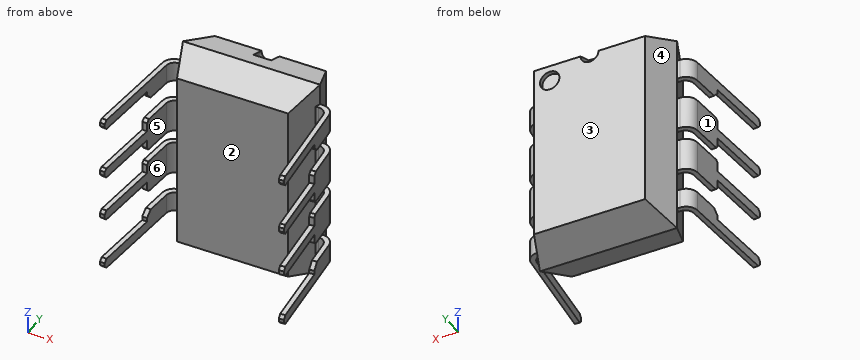
from build123d import *

# Parameters (mm, degrees)
BOSS_EXTRUDE1_DEPTH     = 9.5
CUT_EXTRUDE2_DEPTH      = 9.5
CUT_EXTRUDE2_DEPTH_BACK = 9.5
CUT_EXTRUDE3_DEPTH      = 0.7
SKETCH4_W               = 0.83
SKETCH4_H               = 0.7
CUT_EXTRUDE4_DEPTH      = 0.7
BOSS_EXTRUDE2_START     = -0.762
BOSS_EXTRUDE2_DEPTH     = 0.912
CUT_EXTRUDE5_DEPTH      = 10.15
SKETCH9_R               = 0.45
CUT_EXTRUDE7_DEPTH      = 0.2
BOSS_EXTRUDE3_DEPTH     = 0.762
CUT_EXTRUDE6_DEPTH      = 0.762
MIRROR2_START           = -0.762
MIRROR2_COPY_1_DEPTH    = 0.912
MIRROR2_COPY_2_DEPTH    = 10.15
MIRROR2_COPY_3_DEPTH    = 0.762
MIRROR2_COPY_4_DEPTH    = 0.762


with BuildPart() as part:
    # Sketch1 → Boss-Extrude1 (new body)
    with BuildSketch(Plane.XY):
        Polygon((-24.934327538, -0.557710036), (-25.534514454, 1.091289964), (-30.684140621, 1.091289964), (-31.284327538, -0.557710036), (-30.683412681, -2.208710036), (-25.535242395, -2.208710036), align=None)
    extrude(amount=-BOSS_EXTRUDE1_DEPTH)

    # Sketch2 → Cut-Extrude2 (cut, two sides)
    with BuildSketch(Plane(origin=(-30.683898403, -0.0067685, 0), x_dir=(0, 0, 1), z_dir=(-0.9999999756704636, -0.00022058801540043594, 0))) as cut_extrude2_sk:
        Polygon((-0.616330332, -2.245563479), (0, -0.552209808), (0, -2.212209808), align=None)
        Polygon((-0.60064854, 1.098058491), (0, -0.552209808), (0, 1.098058491), align=None)
        Polygon((-9.5, -2.212209808), (-8.892247033, -2.221997362), (-9.5, -0.552209808), align=None)
        Polygon((-9.5, -0.552209808), (-9.5, 1.098058491), (-8.89935146, 1.098058491), align=None)
    extrude(amount=CUT_EXTRUDE2_DEPTH, mode=Mode.SUBTRACT)
    extrude(cut_extrude2_sk.sketch, amount=-CUT_EXTRUDE2_DEPTH_BACK, mode=Mode.SUBTRACT)

    # Sketch3 → Cut-Extrude3 (cut)
    with BuildSketch(Plane(origin=(0, 1.091289964, 0), x_dir=(1, 0, 0), z_dir=(0, 1, 0))):
        with BuildLine():
            Line((-28.524327536, 0.600475134), (-27.694327539, 0.600408495))
            ThreePointArc((-27.694327539, 0.600408495), (-28.109294218, 1.015441813), (-28.524327536, 0.600475134))
        make_face()
    extrude(amount=-CUT_EXTRUDE3_DEPTH, mode=Mode.SUBTRACT)

    # Sketch4 → Cut-Extrude4 (cut)
    with BuildSketch(Plane(origin=(4.8027e-05, 0, -0.598184984), x_dir=(-0.9999999967769609, 0, -8.028747138262029e-05), z_dir=(8.028747138262029e-05, 0, -0.9999999967769609))):
        with Locations((28.109375655, 0.741289964)):
            Rectangle(SKETCH4_W, SKETCH4_H)
    extrude(amount=-CUT_EXTRUDE4_DEPTH, mode=Mode.SUBTRACT)


with BuildPart() as boss_extrude2_tool:
    # Sketch5 → Boss-Extrude2 (new body)
    with BuildSketch(Plane.XY.offset(-1.143).offset(BOSS_EXTRUDE2_START)):
        with BuildLine():
            Line((-24.934327536, -0.557713614), (-24.80305479, -0.557713614))
            ThreePointArc((-24.80305479, -0.557713614), (-24.431480176, -0.702211079), (-24.255147706, -1.059777956))
            Line((-24.255147706, -1.059777956), (-23.8457982, -5.738664215))
            Line((-23.8457982, -5.738664215), (-24.074922981, -5.758710036))
            Line((-24.074922981, -5.758710036), (-24.477883405, -1.152851317))
            ThreePointArc((-24.477883405, -1.152851317), (-24.606125201, -0.892802679), (-24.876361284, -0.787713614))
            Line((-24.876361284, -0.787713614), (-25.018040872, -0.787713614))
            Line((-25.018040872, -0.787713614), (-24.934327536, -0.557713614))
        make_face()
    boss_extrude2 = extrude(amount=BOSS_EXTRUDE2_DEPTH)


with BuildPart() as part_1:
    add(part.part)


with BuildPart() as part_2:
    # Boss-Extrude2: joined with boss_extrude2_tool
    add(part_1.part.fuse(boss_extrude2_tool.part, tol=0.00001))

    # Sketch6 → Cut-Extrude5 (cut)
    with BuildSketch(Plane(origin=(-24.162916864, -2.113981303, 0), x_dir=(0, 0, -1), z_dir=(0.9961946980917458, 0.08715574274765556, 0))):
        Polygon((0.993, -3.502234692), (0.993, -3.638528611), (1.129293919, -3.638528611), align=None)
        Polygon((1.449, -3.502234692), (1.292810168, -3.638528611), (1.449, -3.638528611), align=None)
        Polygon((1.449, -3.502234692), (1.449, -3.638528611), (1.905, -3.638528611), (1.905, -0.186528611), (1.628, -0.463528611), (1.449, -0.463528611), align=None)
    cut_extrude5 = extrude(amount=-CUT_EXTRUDE5_DEPTH, mode=Mode.SUBTRACT)

    # Sketch9 → Cut-Extrude7 (cut)
    with BuildSketch(Plane(origin=(0, 1.091289964, 0), x_dir=(1, 0, 0), z_dir=(0, 1, 0))):
        with Locations(Location((-26.264514454, 1.330293701, 0), (0, 0, 180))):
            Circle(SKETCH9_R)
    extrude(amount=-CUT_EXTRUDE7_DEPTH, mode=Mode.SUBTRACT)

    # Sketch7 → Boss-Extrude3 (add, symmetric)
    with BuildSketch(Plane.XY.offset(-3.683)):
        with BuildLine():
            Line((-24.934327538, -0.557710036), (-24.803054792, -0.557710036))
            ThreePointArc((-24.803054792, -0.557710036), (-24.431480177, -0.7022075), (-24.255147708, -1.059774377))
            Line((-24.255147708, -1.059774377), (-23.845798202, -5.738660636))
            Line((-23.845798202, -5.738660636), (-24.074922983, -5.758706457))
            Line((-24.074922983, -5.758706457), (-24.477883406, -1.152847739))
            ThreePointArc((-24.477883406, -1.152847739), (-24.606125202, -0.892799101), (-24.876361286, -0.787710036))
            Line((-24.876361286, -0.787710036), (-25.018040873, -0.787710036))
            Line((-25.018040873, -0.787710036), (-24.934327538, -0.557710036))
        make_face()
    boss_extrude3 = extrude(amount=BOSS_EXTRUDE3_DEPTH, both=True)

    # Sketch8 → Cut-Extrude6 (cut)
    with BuildSketch(Plane(origin=(-24.162916555, -2.113981276, 0), x_dir=(0, 0, -1), z_dir=(0.9961946980917459, 0.08715574274765502, 0))):
        Polygon((2.921, -3.638525046), (3.4545, -3.638525046), (3.4545, -3.512139824), (3.4545, -0.463528611), (3.048, -0.463528611), (2.921, -0.309075706), align=None)
        Polygon((3.9115, -0.463528611), (3.9115, -3.512139824), (3.9115, -3.638525046), (4.445, -3.638525046), (4.445, -0.359101958), (4.318, -0.463528611), align=None)
        Polygon((3.4545, -3.512139824), (3.4545, -3.638525046), (3.558421148, -3.638525046), align=None)
        Polygon((3.9115, -3.512139824), (3.757794765, -3.638525046), (3.9115, -3.638525046), align=None)
    cut_extrude6 = extrude(amount=-CUT_EXTRUDE6_DEPTH, mode=Mode.SUBTRACT)

    # Mirror1: Boss-Extrude2, Cut-Extrude5, Boss-Extrude3, Cut-Extrude6 across plane
    add(boss_extrude2.mirror(Plane.XY.offset(-4.75)))
    add(cut_extrude5.mirror(Plane.XY.offset(-4.75)), mode=Mode.SUBTRACT)
    add(boss_extrude3.mirror(Plane.XY.offset(-4.75)))
    add(cut_extrude6.mirror(Plane.XY.offset(-4.75)), mode=Mode.SUBTRACT)

    # Mirror2: Boss-Extrude2, Cut-Extrude5, Boss-Extrude3, Cut-Extrude6 across plane
    add(boss_extrude2.mirror(Plane(origin=(-28.109327538, 0, 0), x_dir=(0, 0, 1), z_dir=(1, 0, 0))))
    add(cut_extrude5.mirror(Plane(origin=(-28.109327538, 0, 0), x_dir=(0, 0, 1), z_dir=(1, 0, 0))), mode=Mode.SUBTRACT)
    add(boss_extrude3.mirror(Plane(origin=(-28.109327538, 0, 0), x_dir=(0, 0, 1), z_dir=(1, 0, 0))))
    add(cut_extrude6.mirror(Plane(origin=(-28.109327538, 0, 0), x_dir=(0, 0, 1), z_dir=(1, 0, 0))), mode=Mode.SUBTRACT)


with BuildPart() as mirror2_copy_1_tool:
    # Mirror2 copy 1 sketch → Mirror2 copy 1 (new body)
    with BuildSketch(Plane(origin=(-56.218655076, 0, -8.357), x_dir=(-1, 0, 0), z_dir=(0, 0, -1)).offset(MIRROR2_START)):
        with BuildLine():
            Line((-24.934327536, -0.557713614), (-24.80305479, -0.557713614))
            ThreePointArc((-24.80305479, -0.557713614), (-24.431480176, -0.702211079), (-24.255147706, -1.059777956))
            Line((-24.255147706, -1.059777956), (-23.8457982, -5.738664215))
            Line((-23.8457982, -5.738664215), (-24.074922981, -5.758710036))
            Line((-24.074922981, -5.758710036), (-24.477883405, -1.152851317))
            ThreePointArc((-24.477883405, -1.152851317), (-24.606125201, -0.892802679), (-24.876361284, -0.787713614))
            Line((-24.876361284, -0.787713614), (-25.018040872, -0.787713614))
            Line((-25.018040872, -0.787713614), (-24.934327536, -0.557713614))
        make_face()
    extrude(amount=MIRROR2_COPY_1_DEPTH)


with BuildPart() as part_3:
    add(part_2.part)


with BuildPart() as part_4:
    # Mirror2 copy 1: joined with mirror2_copy_1_tool
    add(part_3.part.fuse(mirror2_copy_1_tool.part, tol=0.00001))

    # Mirror2 copy 2 sketch → Mirror2 copy 2 (cut)
    with BuildSketch(Plane(origin=(-32.055738211, -2.113981303, -9.5), x_dir=(0, 0, 1), z_dir=(-0.9961946980917458, 0.08715574274765556, 0))):
        Polygon((0.993, -3.502234692), (0.993, -3.638528611), (1.129293919, -3.638528611), align=None)
        Polygon((1.449, -3.502234692), (1.292810168, -3.638528611), (1.449, -3.638528611), align=None)
        Polygon((1.449, -3.502234692), (1.449, -3.638528611), (1.905, -3.638528611), (1.905, -0.186528611), (1.628, -0.463528611), (1.449, -0.463528611), align=None)
    extrude(amount=-MIRROR2_COPY_2_DEPTH, mode=Mode.SUBTRACT)

    # Mirror2 copy 3 sketch → Mirror2 copy 3 (add, symmetric)
    with BuildSketch(Plane(origin=(-56.218655076, 0, -5.817), x_dir=(-1, 0, 0), z_dir=(0, 0, -1))):
        with BuildLine():
            Line((-24.934327538, -0.557710036), (-24.803054792, -0.557710036))
            ThreePointArc((-24.803054792, -0.557710036), (-24.431480177, -0.7022075), (-24.255147708, -1.059774377))
            Line((-24.255147708, -1.059774377), (-23.845798202, -5.738660636))
            Line((-23.845798202, -5.738660636), (-24.074922983, -5.758706457))
            Line((-24.074922983, -5.758706457), (-24.477883406, -1.152847739))
            ThreePointArc((-24.477883406, -1.152847739), (-24.606125202, -0.892799101), (-24.876361286, -0.787710036))
            Line((-24.876361286, -0.787710036), (-25.018040873, -0.787710036))
            Line((-25.018040873, -0.787710036), (-24.934327538, -0.557710036))
        make_face()
    extrude(amount=MIRROR2_COPY_3_DEPTH, both=True)

    # Mirror2 copy 4 sketch → Mirror2 copy 4 (cut)
    with BuildSketch(Plane(origin=(-32.055738521, -2.113981276, -9.5), x_dir=(0, 0, 1), z_dir=(-0.9961946980917459, 0.08715574274765502, 0))):
        Polygon((2.921, -3.638525046), (3.4545, -3.638525046), (3.4545, -3.512139824), (3.4545, -0.463528611), (3.048, -0.463528611), (2.921, -0.309075706), align=None)
        Polygon((3.9115, -0.463528611), (3.9115, -3.512139824), (3.9115, -3.638525046), (4.445, -3.638525046), (4.445, -0.359101958), (4.318, -0.463528611), align=None)
        Polygon((3.4545, -3.512139824), (3.4545, -3.638525046), (3.558421148, -3.638525046), align=None)
        Polygon((3.9115, -3.512139824), (3.757794765, -3.638525046), (3.9115, -3.638525046), align=None)
    extrude(amount=-MIRROR2_COPY_4_DEPTH, mode=Mode.SUBTRACT)


solid = part_4.part
Source: CAD feature listing. Evaluate the final solid. Frame: model axes, mm. Face numbers are marked on the shaded views. A direction names the side the tool comes from. Round coordinates to 2 decimals unless told otherwise and drop trailing zeros. Loops run counter-clockwise (first coordinate to the right, second up) from the corner with the lowest first, then second, coordinate; pieces in that order, holes last. Notation, with made-up numbers: (88, 14.5) - (145, 14.5) arc R28 cw to (145, 42.5) - close; hole circle Ø8 at (89, 55). An arc over 180 degrees is marked (long way). Write item = value, one per line. Start each with the question number.
Item 1: Mould query, pull axis X, two halves, no side actions, for the marked faces 3, 4, 5 and 6. Classes: released by +X, released by -X, zero draft, split by the parting line, or undercut.
Item 2: Section query A-A on y = -4.25. Count the separate pieces of the cut face and the enclosed holes in it, plus the area to 3 significant figures.
Item 3: First-contact query: pin 1 Ø1 at (y, z) = (-2.5, -5) entering from +X; pin 2 Ø1.5 at (x, z) = (-28.5, -4.5) entering from -Y; pin 3 Ø1 at (x, y) = (-31.5, -2) entering from -Z. Flat tips, straight axial feed; report the tip coordinate or a pass-through.
Item 4: Section query B-B on z = -8.75. Output: boundary loops of the cut face in (x, y), plus the area to 3 significant figures.
Item 5: Reachability of the marked faces 1 and 2 from +Z, -Z, +X, -X, +Y, -Y: full face, straight path, thin tool, end or side. Return the list, or none.
Item 6: Material intervals for line 1 (X direction, y = -1.75, z = -8.25); line 2 (Y direction, x = -27.75, z = -5); line 3 (Y direction, x = -28.25, z = -0.75), sorted ascending.
Item 7: Section query C-C on x = -27. Output: boundary loops of the cut face in (y, z).
Results list:
q1.face_3 = zero draft
q1.face_4 = released by -X
q1.face_5 = undercut
q1.face_6 = undercut
q2.separate_pieces = 8
q2.enclosed_holes = 0
q2.area = 0.843 mm²
q3.pin_1 = -24.12
q3.pin_2 = -2.21
q3.pin_3 = -8.51
q4.outline = (-31.28, -0.56) - (-30.68, -2.21) - (-25.54, -2.21) - (-24.93, -0.56) - (-25.53, 1.09) - (-30.68, 1.09) - close
q4.area = 19.0 mm²
q5.face_1 = +Z, -Z, -X, +Y
q5.face_2 = +Z, -Z, -Y
q6.line_1 = -32.02 to -31.79, -30.85 to -25.37, -24.43 to -24.19
q6.line_2 = -2.21 to 1.09
q6.line_3 = -2.21 to 0.39
q7.outline = (-2.21, -8.9) - (-0.56, -9.5) - (1.09, -8.9) - (1.09, -0.6) - (-0.56, 0) - (-2.21, -0.6) - close
